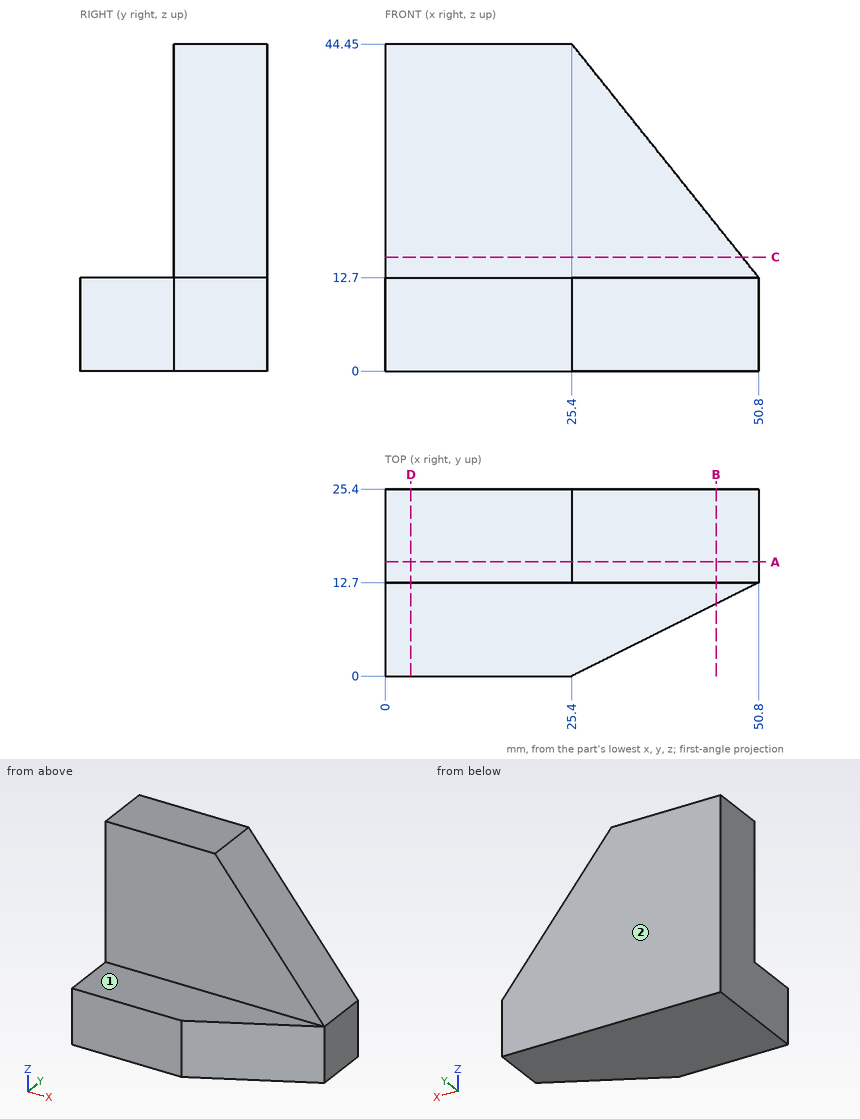
Check sheet for the drawn part. Datum: minimum x, y, z corner. Units: mm. A direction names the side the tool comes from. Give positions to 0.01 mm unless a question says otherwise; leave off trailing zeros. Order: outer loops, then holes, each group sorted by start corner. A loop starts at its lowest first (then second) coordinate and runs counter-clockwise, first axis right, second up. Notation, with made-up numbers: (-38, -24.75) -> (-27, -24.75) arc R25 ccw to (-27, 13.25) -> close; hole circle Ø11 at (-15.5, -20). An arc over 180 degrees is marked (long way). Use a Markdown table: item, result.
1) Section check D-D, the plane x = 3.5. Record the boundary of the cut face in (y, z), then the cut area to 3 significant figures.
Results:
| item | result |
|---|---|
| outline | (0, 0) -> (25.4, 0) -> (25.4, 44.45) -> (12.7, 44.45) -> (12.7, 12.7) -> (0, 12.7) -> close |
| area | 726 mm² |
2) Tool access check on the marked faces 1 and 2. Record the directions out of +Z, -Z, +X, -X, +Y, -Y that give a thin tool (end or side, any length) a straight path to the whole face; none if there is none.
Results:
| item | result |
|---|---|
| face 1 | +Z, +X, -X, -Y |
| face 2 | +Z, -Z, +X, -X, +Y |
3) Depth check by flat-ended pin: pin 1 Ø12 at (x, z) = (26, 25) entering from -Y; pin 2 Ø4 at (x, y) = (37.5, 5) entering from +Z; pin 3 Ø5 at (y, z) = (10, 11) entering from +X. Enter the tip coordinate at first touch or a pass-through.
Results:
| item | result |
|---|---|
| pin 1 | y = 12.7 |
| pin 2 | z = 12.7 |
| pin 3 | x = 50.4 |
4) Section check C-C, the plane z = 15.5. Record the boundary of the cut face in (x, y), then the cut area to 3 significant figures.
Results:
| item | result |
|---|---|
| outline | (0, 12.7) -> (48.56, 12.7) -> (48.56, 25.4) -> (0, 25.4) -> close |
| area | 617 mm² |
5) Section check A-A, the plane y = 15.5. Record the boundary of the cut face in (x, z), then the cut area to 3 significant figures.
Results:
| item | result |
|---|---|
| outline | (0, 0) -> (50.8, 0) -> (50.8, 12.7) -> (25.4, 44.45) -> (0, 44.45) -> close |
| area | 1,850 mm² |
6) Material ranges on probe 1 along Z at (x, y) = (5.5, 2.5); probe 2 along Y at (x, z) = (6, 40.5); probe 3 along X at (y, z) = (23.25, 23.5), recorded low to high.
Results:
| item | result |
|---|---|
| probe 1 | 0 to 12.7 |
| probe 2 | 12.7 to 25.4 |
| probe 3 | 0 to 42.16 |
7) Section check B-B, the plane x = 45. Record the boundary of the cut face in (y, z), then the cut area to 3 significant figures.
Results:
| item | result |
|---|---|
| outline | (9.8, 0) -> (25.4, 0) -> (25.4, 19.95) -> (12.7, 19.95) -> (12.7, 12.7) -> (9.8, 12.7) -> close |
| area | 290 mm² |
